Input: part model. Units: mm. Frame: model coordinates. Face numbers are marked on the shaded views. A direction names the side the tool comes from. Coordinates: 2 decimals unless noted, no trailing zeros. Loops run counter-clockwise (first coordinate to the right, second up) from the corner with the lowest first, then second, coordinate; pieces in that order, holes last.
```python
from build123d import *

# Parameters (mm, degrees)
SKETCH1_R           = 5.5
BOSS_EXTRUDE1_DEPTH = 16
SKETCH2_R           = 3.5
BOSS_EXTRUDE2_DEPTH = 1
SKETCH3_R           = 5.5
BOSS_EXTRUDE3_DEPTH = 1
SKETCH5_W           = 1
SKETCH5_H           = 4
FILLET1_R           = 2
BOSS_EXTRUDE4_DEPTH = 3
SKETCH8_R           = 3.5
BOSS_EXTRUDE5_DEPTH = 3
BOSS_EXTRUDE7_DEPTH = 1
SKETCH17_R          = 2.5
CUT_EXTRUDE7_DEPTH  = 6
SKETCH18_R          = 1.25
CUT_EXTRUDE8_DEPTH  = 26.129663746
SKETCH19_R          = 4.5
CUT_EXTRUDE9_DEPTH  = 1.5
SKETCH21_R          = 3
CUT_EXTRUDE10_DEPTH = 30.314547048
CUT_EXTRUDE12_DEPTH = 3
SKETCH24_R          = 1
CUT_EXTRUDE13_DEPTH = 3


with BuildPart() as part:
    # Sketch1 → Boss-Extrude1 (new body)
    with BuildSketch(Plane(origin=(0, 0, 0), x_dir=(0, 0, -1), z_dir=(1, 0, 0))):
        Circle(SKETCH1_R)
    extrude(amount=BOSS_EXTRUDE1_DEPTH)

    # Sketch2 → Boss-Extrude2 (add)
    with BuildSketch(Plane(origin=(16, 0, 0), x_dir=(0, 0, -1), z_dir=(1, 0, 0))):
        Circle(SKETCH2_R)
    extrude(amount=BOSS_EXTRUDE2_DEPTH)

    # Sketch3 → Boss-Extrude3 (add)
    with BuildSketch(Plane(origin=(17, 0, 0), x_dir=(0, 0, -1), z_dir=(1, 0, 0))):
        Circle(SKETCH3_R)
    extrude(amount=BOSS_EXTRUDE3_DEPTH)

    # Sweep1: sweep along a path in Sketch4
    with BuildLine(Plane(origin=(0, 0, 0), x_dir=(1, 0, 0), z_dir=(0, 1, 0))) as sweep1_path:
        Line((25.5, 15.5), (25.5, 7.5))
        ThreePointArc((25.5, 7.5), (25.207106781, 6.792893219), (24.5, 6.5))
        Line((24.5, 6.5), (18.5, 6.5))
        ThreePointArc((18.5, 6.5), (17.792893219, 6.207106781), (17.5, 5.5))
        Line((17.5, 5.5), (17.5, 4.331461844))
    # Sketch5 → Sweep1 (sweep)
    with BuildSketch(Plane.XY.offset(-15.5)):
        with Locations((25.5, 0)):
            Rectangle(SKETCH5_W, SKETCH5_H)
    sweep(path=sweep1_path.line)

    # Fillet1
    fillet1_edges = [part.edges().sort_by_distance(p)[0] for p in [
        (25.5, -2, -15.5),
        (25.5, 2, -15.5),
    ]]
    fillet(fillet1_edges, radius=FILLET1_R - 0.0001)  # a hair under: the kernel refuses the full size

    # Sketch7 → Boss-Extrude4 (add)
    with BuildSketch(Plane(origin=(18, 0, 0), x_dir=(0, 0, -1), z_dir=(1, 0, 0))):
        Polygon((-2.020725942, -3.5), (2.020725942, -3.5), (4.041451884, 0), (2.020725942, 3.5), (-2.020725942, 3.5), (-4.041451884, 0), align=None)
    extrude(amount=BOSS_EXTRUDE4_DEPTH)

    # Sketch8 → Boss-Extrude5 (add)
    with BuildSketch(Plane(origin=(21, 0, 0), x_dir=(0, 0, -1), z_dir=(1, 0, 0))):
        Circle(SKETCH8_R)
    extrude(amount=BOSS_EXTRUDE5_DEPTH)

    # Sketch9 → Boss-Extrude7 (add)
    with BuildSketch(Plane(origin=(24, 0, 0), x_dir=(0, 0, -1), z_dir=(1, 0, 0))):
        Polygon((-2.020725942, -3.5), (2.020725942, -3.5), (4.041451884, 0), (2.020725942, 3.5), (-2.020725942, 3.5), (-4.041451884, 0), align=None)
    extrude(amount=BOSS_EXTRUDE7_DEPTH)

    # Sketch17 → Cut-Extrude7 (cut)
    with BuildSketch(Plane(origin=(25, 0, 0), x_dir=(0, 0, -1), z_dir=(1, 0, 0))):
        Circle(SKETCH17_R)
    extrude(amount=-CUT_EXTRUDE7_DEPTH, mode=Mode.SUBTRACT)

    # Sketch18 → Cut-Extrude8 (cut, through all)
    with BuildSketch(Plane(origin=(19, 0, 0), x_dir=(0, 0, -1), z_dir=(1, 0, 0))):
        Circle(SKETCH18_R)
    extrude(amount=-CUT_EXTRUDE8_DEPTH, mode=Mode.SUBTRACT)

    # Sketch19 → Cut-Extrude9 (cut)
    with BuildSketch(Plane.ZY):
        Circle(SKETCH19_R)
    extrude(amount=-CUT_EXTRUDE9_DEPTH, mode=Mode.SUBTRACT)

    # Sketch21 → Cut-Extrude10 (cut, through all)
    with BuildSketch(Plane(origin=(0, -2.75, -4.763139721), x_dir=(-1, 0, 0), z_dir=(0, -0.5000000000000002, -0.8660254037844385))):
        with Locations(Location((-5.001832393, 0.406031974, 0), (0, 0, 90))):
            Circle(SKETCH21_R)
    extrude(amount=-CUT_EXTRUDE10_DEPTH, mode=Mode.SUBTRACT)

    # Sketch23 → Cut-Extrude12 (cut)
    with BuildSketch(Plane(origin=(0, 5.5, 0), x_dir=(1, 0, 0), z_dir=(0, 1, 0))):
        Polygon((11, 5.5), (13.5, -5.5), (11.5, -5.5), (9, 5.5), align=None)
    extrude(amount=-CUT_EXTRUDE12_DEPTH, mode=Mode.SUBTRACT)

    # Sketch24 → Cut-Extrude13 (cut)
    with BuildSketch(Plane.ZY.offset(-25)):
        with Locations((-13.5, 0)):
            Circle(SKETCH24_R)
        with Locations((-10.5, 0)):
            Circle(SKETCH24_R)
    extrude(amount=-CUT_EXTRUDE13_DEPTH, mode=Mode.SUBTRACT)


solid = part.part
```
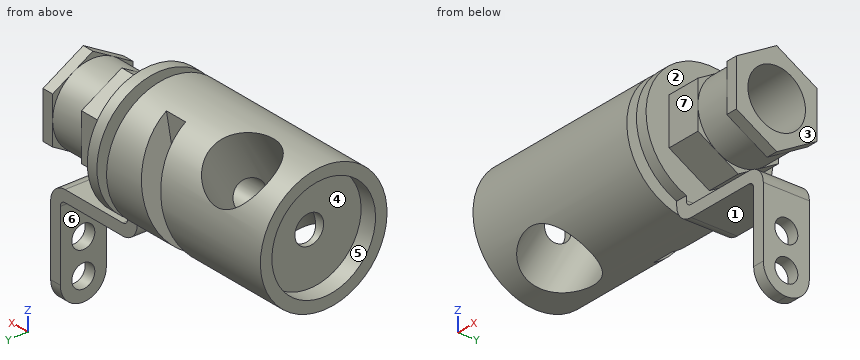
Item 1: Mould query, pull axis Z, two halves, no side actions, for the marked faces 1, 2, 3 and 4. Classes: +Z half, -Z half, draft (parallel to the pull), parting line (faces both ways), or undercut.
Result:
face 1: -Z half
face 2: undercut
face 3: draft
face 4: undercut
Item 2: Section query C-C (x = 13.75). Output: boundary loops of the cut face in (y, z).
Result:
outline: circle Ø11 at (0, 0); hole circle Ø2.5 at (0, 0)
Item 3: Line query: L1, parallel to X at y = 1.25, z = 1.5; L2, parallel to Y at x = 25.75, z = -13.5; L3, parallel to X at y = -4.75, z = 1. Output: solid intervals per line, ascending.
Result:
L1: x = 1.5 to 2, 8 to 19
L2: y = -2 to -1, 1 to 2
L3: x = 0 to 16, 17 to 18
Item 4: Contact query for flat-ended pins moving along their axis: P1, Ø6, axis at y = 0, z = 0, coming from the -X side; P2, Ø1.5, axis at x = 6.5, y = -3.5, coming from the +Z side; P3, Ø0.8, axis at y = 1, z = 3.5, coming from the +X side; P4, Ø1.2, axis at y = 0, z = -10.5, coming from the +X side. Output: stop coordinate, or through.
Result:
P1: stops at x = 1.5
P2: stops at z = 4.76
P3: stops at x = 25
P4: passes through
Item 5: Reachability of the marked faces 5, 6 and 7 from +Z, -Z, +X, -X, +Y, -Y: full face, straight path, thin tool, end or side. Return the list, or none.
Result:
face 5: -X
face 6: -Z, -X, +Y, -Y
face 7: +Z, -Z, +X, -Y
Item 6: Section query A-A (x = 22.25). Output: boundary loops of the cut face in (y, z).
Result:
outline: circle Ø7 at (0, 0); (-2, -7) - (2, -7) - (2, -6) - (-2, -6) - close; hole circle Ø5 at (0, 0)
Item 7: Section query B-B (z = -10.5). Output: boundary loops of the cut face in (x, y), then the cut area to 3 significant figures.
Result:
outline: (25, -2) - (26, -2) - (26, -1) - (25, -1) - close; (25, 1) - (26, 1) - (26, 2) - (25, 2) - close
area: 2.00 mm2
Item 8: Section query D-D (x = 4.5). Output: boundary loops of the cut face in (y, z).
Result:
outline: (-4.65, -2.94) - (0.23, 5.5) arc R5.5 ccw to start; (0.74, -5.45) arc R5.5 ccw to (5.09, 2.09) - close
